Design review of the part shown in the three views and the two pictorial views. Dimensions are in mm from the part's minimum x, y and z. A direction names the side the tool comes from. Coordinates: 2 decimals unless noted, no trailing zeros. Loops run counter-clockwise (first coordinate to the right, second up) from the corner with the lowest first, then second, coordinate; pieces in that order, holes last. Notation, with made-up numbers: (80, -13.5) -> (133, -13.5) arc R15 cw to (133, -2.5) -> close; hole circle Ø5 at (70, -27.5). An arc over 180 degrees is marked (long way). One line per item, written item: value.
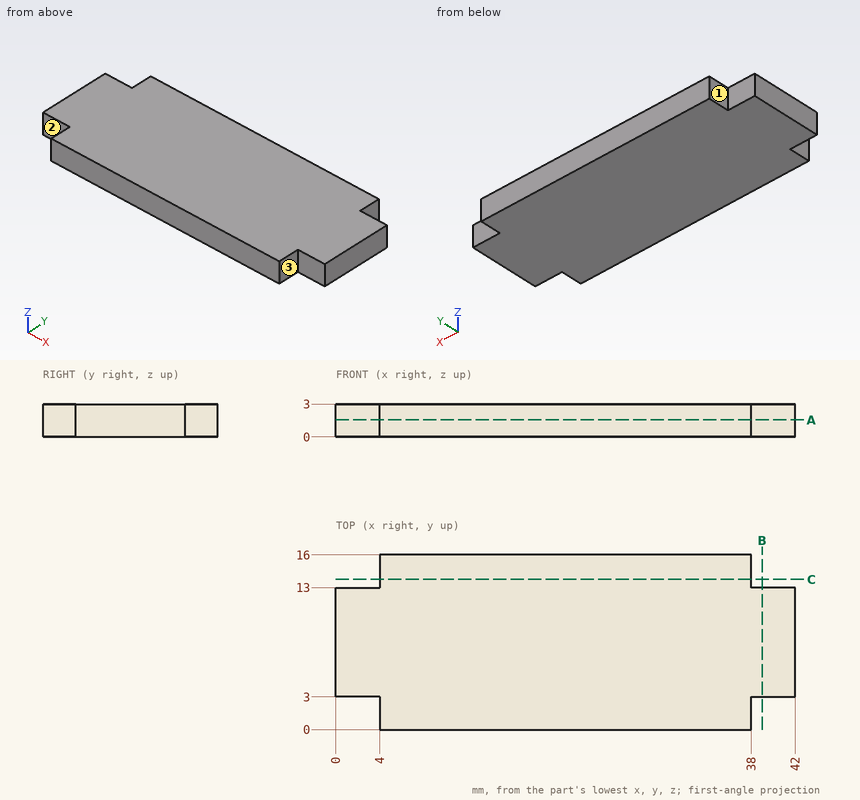
1. Take a section at A-A, the plane z = 1.55. Give the boundary of the cut face in (x, y).
Return value:
outline: (0, 3) -> (4, 3) -> (4, 0) -> (38, 0) -> (38, 3) -> (42, 3) -> (42, 13) -> (38, 13) -> (38, 16) -> (4, 16) -> (4, 13) -> (0, 13) -> close
2. Take a section at C-C, the plane y = 13.75. Give the boundary of the cut face in (x, z), and give its area (3 significant figures).
Return value:
outline: (4, 0) -> (38, 0) -> (38, 3) -> (4, 3) -> close
area: 102 mm2
3. To check wall thickness, follow probe 1 along X at (y, z) = (13.5, 1.3); probe 2 along Y at (x, z) = (40, 0.9). State the ranges of each line that lie inside material, in increasing order. Write a range as from..to.
Return value:
probe 1: x = 4..38
probe 2: y = 3..13
4. Take a section at B-B, the plane x = 39. Give the boundary of the cut face in (y, z), and give its area (3 significant figures).
Return value:
outline: (3, 0) -> (13, 0) -> (13, 3) -> (3, 3) -> close
area: 30.0 mm2
5. For the marked faces 1, 2 and 3, list the 3-axis set-ups (+Z, -Z, +X, -X, +Y, -Y) from which the entire face can be reached by the end or side of a thin tool; tool diameter is ignored.
Return value:
face 1: +Z, -Z, -X, +Y
face 2: +Z, -Z, -X, -Y
face 3: +Z, -Z, +X, -Y
6. Insertion check: pin 1 Ø1.5 at (y, z) = (14.5, 2) entering from +X. The pin has a flat end and moves straight along its axis. Give the tip position at first contact, or say it passes through.
Return value:
pin 1: stops at x = 38
